Here's how the part is built. I have some questions about the finished solid (model axes, mm). A direction names the side the tool comes from. Coordinates: 2 decimals unless noted, no trailing zeros. Write each loop counter-clockwise with the first axis right and the second up, starting at its lowest first coordinate (ties: lowest second). Pieces come first, ordered by that corner, then holes. Notation, with made-up numbers: (36.5, 81) - (44.5, 81) arc R21 cw to (44.5, 116) - close; hole circle Ø2 at (45, 68.25). An arc over 180 degrees is marked (long way). Answer in a Markdown table with one row per item. Add a question column.
Item 1: If I drill on probe 1 along X at (y, z) = (-11, -10); probe 2 along Y at (x, z) = (-11, -6.5); probe 3 along X at (y, z) = (11, -6), over which ranges is the centre line in solid material (lowest first)? Write a range as from..to.
Item 2: I'm going to push flat-ended pins straight in: pin 1 (2 mm diameter, centred on y = -11, z = -5, fed in from +X); pin 2 (5 mm diameter, centred on y = -6, z = -5.5, fed in from +X); pin 3 (10 mm diameter, centred on x = -22.5, y = 5, fed in from +Z). Where does each tip first touch, or does it pass through?
Item 3: Imagine slicing it at B-B (y = 0). Please give me the cut outline in (x, z).
Item 4: We'd pull the mould along X, two halves only. Please class faces 1 (the face through (-2.17, -9.76, 1.48)), 2 (the face through (-28, 3, 0.1)), 3 (the face through (4.368, -11.514, -3.866)): +X half, -X half, draft (parallel to the pull), parting line (faces both ways), or undercut.
Item 5: Imagine slicing it at D-D (z = -11.5). Please give me the cut outline in (x, y).
Item 6: Imagine slicing it at C-C (z = -1.75). Please give me the cut outline in (x, y), plus the area to 3 significant figures.
Item 7: Which directions (+Z, -Z, +X, -X, +Y, -Y) give clear straight access to the entire face, cutting with the end or side of a thin tool? Please do faces 4 (the face through (-8, -7, 0)), 5 (the face through (-8, 12, -7.855)), 6 (the face through (-9.765, -12, -5)), 7 (the face through (-24, 0, -2.9)).
Item 8: Imagine slicing it at A-A (x = 0). Please give me the cut outline in (y, z), plus the area to 3 significant figures.
from build123d import *

# Parameters (mm, degrees)
SKETCH_1_W          = 24.561403508
SKETCH_1_H          = 25
SKETCH_1_R          = 10
EXTRUDE_1_DEPTH     = 3
EXTRUDE_START       = -2.9
SKETCH_2_W          = 29
SKETCH_2_H          = 25
EXTRUDE_2_DEPTH     = 3
SKETCH_4_W          = 2
SKETCH_4_H          = 25
EXTRUDE_3_DEPTH     = 10
EXTRUDE_4_DEPTH     = 2
SKETCH_6_R          = 1.2
EXTRUDE_5_DEPTH     = 2
SKETCH_7_R          = 2
CUT_EXTRUDE_1_DEPTH = 45.275798551
FILLET_1_R          = 3


with BuildPart() as part:
    # Эскиз1 → Бобышка-Вытянуть1 (new body)
    with BuildSketch(Plane.XY):
        Rectangle(SKETCH_1_W, SKETCH_1_H)
        Circle(SKETCH_1_R, mode=Mode.SUBTRACT)
    extrude(amount=EXTRUDE_1_DEPTH)

    # Эскиз2 → Бобышка-Вытянуть2 (add)
    with BuildSketch(Plane.XY.offset(3).offset(EXTRUDE_START)):
        with Locations((-26.780701754, 0)):
            Rectangle(SKETCH_2_W, SKETCH_2_H)
    extrude(amount=-EXTRUDE_2_DEPTH)

    # Эскиз4 → Бобышка-Вытянуть3 (add)
    with BuildSketch(Plane(origin=(0, 0, -2.9), x_dir=(-1, 0, 0), z_dir=(0, 0, -1))):
        with Locations((13.280701754, 0)):
            Rectangle(SKETCH_4_W, SKETCH_4_H)
        with Locations((40.280701754, 0)):
            Rectangle(SKETCH_4_W, SKETCH_4_H)
    extrude(amount=EXTRUDE_3_DEPTH)

    # Эскиз5 → Бобышка-Вытянуть4 (add)
    with BuildSketch(Plane(origin=(0, 12.5, 0), x_dir=(1, 0, 0), z_dir=(0, 1, 0))):
        Polygon((-14.280701754, 7.855101529), (-14.280701754, -0.1), (-12.280701754, -0.1), (-12.280701754, -3), (12.280701754, -3), (12.280701754, 0), (-3.796991433, 7.855101529), align=None)
    extrude(amount=-EXTRUDE_4_DEPTH)

    # Эскиз6 → Бобышка-Вытянуть5 (add)
    with BuildSketch(Plane.XZ.offset(12.5)):
        with BuildLine():
            Line((-12.280701754, 0), (-12.280701754, -7.855101529))
            Line((-12.280701754, -7.855101529), (-10.765310979, -7.855101529))
            ThreePointArc((-10.765310979, -7.855101529), (-10.058204198, -7.56220831), (-9.765310979, -6.855101529))
            Line((-9.765310979, -6.855101529), (-9.765310979, -2.916331119))
            ThreePointArc((-9.765310979, -2.916331119), (-7.265310979, -0.416331119), (-4.765310979, -2.916331119))
            Line((-4.765310979, -2.916331119), (-4.765310979, -6.726653445))
            ThreePointArc((-4.765310979, -6.726653445), (-4.294942972, -7.574880981), (-3.326331075, -7.625150325))
            Line((-3.326331075, -7.625150325), (12.280701754, 0))
            Line((12.280701754, 0), (-12.280701754, 0))
        make_face()
        with Locations(Location((-2.663311188, -4.066950409, 0), (0, 0, 270))):
            Circle(SKETCH_6_R, mode=Mode.SUBTRACT)
    extrude(amount=-EXTRUDE_5_DEPTH)

    # Эскиз7 → Вырез-Вытянуть1 (cut, through all)
    with BuildSketch(Plane(origin=(0, 0, -2.9), x_dir=(-1, 0, 0), z_dir=(0, 0, -1))):
        with Locations((26.780701754, 0)):
            Circle(SKETCH_7_R)
    extrude(amount=-CUT_EXTRUDE_1_DEPTH, mode=Mode.SUBTRACT)

    # Скругление1
    # the kernel refuses this fillet: 3 mm, written as the material it adds along each edge
    with BuildSketch(Plane(origin=(-12.280701754, -12.5, 0.1), x_dir=(0, 0, 1), z_dir=(0, 1, 0))) as fillet_1_piece_1:
        with BuildLine():
            CenterArc((3, -2.99833287), FILLET_1_R, 91.910213172, 88.089786828)
            Line((0, -2.99833287), (-0.06, -2.99833287))
            Line((-0.06, -2.99833287), (-0.06, 0))
            Line((-0.06, 0), (0, 0.06))
            ThreePointArc((0, 0.06), (1.45, 0.06), (2.898, 0.059966657))
            Line((2.898, 0.059966657), (2.9, 0))
        make_face()
    extrude(amount=25)


solid = part.part
Here are the results:
| question | item | result |
|---|---|---|
| 1 | probe 1 | x = -41.28..-39.28, -14.28..-12.28 |
| 1 | probe 2 | y = -12.5..-10.5, 10.5..12.5 |
| 1 | probe 3 | x = -41.28..-39.28, -14.28..0 |
| 2 | pin 1 | stops at x = 4.09 |
| 2 | pin 2 | stops at x = -12.28 |
| 2 | pin 3 | stops at z = 0.1 |
| 3 | outline | (-41.28, -12.9) - (-39.28, -12.9) - (-39.28, -2.9) - (-28.78, -2.9) - (-28.78, 0.1) - (-41.28, 0.1) - close; (-24.78, -2.9) - (-14.28, -2.9) - (-14.28, -12.9) - (-12.28, -12.9) - (-12.28, 0) - (-10, 0) - (-10, 3) - (-12.28, 3) arc R3 cw to (-15.28, 0.1) - (-24.78, 0.1) - close; (10, 0) - (12.28, 0) - (12.28, 3) - (10, 3) - close |
| 4 | face 1 | undercut |
| 4 | face 2 | draft |
| 4 | face 3 | +X half |
| 5 | outline | (-41.28, -12.5) - (-39.28, -12.5) - (-39.28, 12.5) - (-41.28, 12.5) - close; (-14.28, -12.5) - (-12.28, -12.5) - (-12.28, 12.5) - (-14.28, 12.5) - close |
| 6 | outline | (-41.28, -12.5) - (-9.48, -12.5) - (-9.48, -10.5) - (-12.28, -10.5) - (-12.28, 10.5) - (8.7, 10.5) - (8.7, 12.5) - (-41.28, 12.5) - close; (-5.05, -12.5) - (8.7, -12.5) - (8.7, -10.5) - (-5.05, -10.5) - close; hole circle Ø4 at (-26.78, 0) |
| 6 | area | 788 mm2 |
| 7 | face 4 | -Z, +X |
| 7 | face 5 | -Z, +X, +Y, -Y |
| 7 | face 6 | -Z, -Y |
| 7 | face 7 | -Z, +Y, -Y |
| 8 | outline | (-12.5, -6) - (-10.5, -6) - (-10.5, 0) - (-10, 0) - (-10, 3) - (-12.5, 3) - close; (10, 0) - (10.5, 0) - (10.5, -6) - (12.5, -6) - (12.5, 3) - (10, 3) - close |
| 8 | area | 39.0 mm2 |
